```python
from build123d import *

# Parameters (mm, degrees)
SKETCH1_W           = 19
SKETCH1_H           = 81
BOSS_EXTRUDE1_DEPTH = 12.5
SKETCH2_W           = 8.5
SKETCH2_H           = 81
CUT_EXTRUDE1_DEPTH  = 6
SKETCH3_W           = 31.784398885
SKETCH3_H           = 20.084620154
CUT_EXTRUDE2_DEPTH  = 82.482700732
SKETCH4_W           = 27.793270948
SKETCH4_H           = 17.497219338
CUT_EXTRUDE3_DEPTH  = 82.444960882
SKETCH5_W           = 2
SKETCH5_H           = 6.3
BOSS_EXTRUDE2_DEPTH = 6


with BuildPart() as part:
    # Sketch1 → Boss-Extrude1 (new body)
    with BuildSketch(Plane.XY):
        with Locations((-0.214285714, -27.308823529)):
            Rectangle(SKETCH1_W, SKETCH1_H)
    extrude(amount=BOSS_EXTRUDE1_DEPTH)

    # Sketch2 → Cut-Extrude1 (cut)
    with BuildSketch(Plane(origin=(0, 0, 0), x_dir=(-1, 0, 0), z_dir=(0, 0, -1))):
        with Locations((0.214285714, -27.308823529)):
            Rectangle(SKETCH2_W, SKETCH2_H)
    extrude(amount=-CUT_EXTRUDE1_DEPTH, mode=Mode.SUBTRACT)

    # Sketch3 → Cut-Extrude2 (cut, through all)
    with BuildSketch(Plane(origin=(0, -64.772690644, -9.103208009), x_dir=(1, 0, 0), z_dir=(0, -0.9902680687415703, -0.13917310096006574))):
        with Locations((-0.737280551, 17.487835558)):
            Rectangle(SKETCH3_W, SKETCH3_H)
    extrude(amount=CUT_EXTRUDE2_DEPTH, mode=Mode.SUBTRACT)

    # Sketch4 → Cut-Extrude3 (cut, through all)
    with BuildSketch(Plane(origin=(0, 12.138481454, 12.138481454), x_dir=(-1, 0, 0), z_dir=(0, 0.7071067811865464, 0.7071067811865488))):
        with Locations((0.087709147, -6.370587608)):
            Rectangle(SKETCH4_W, SKETCH4_H)
    extrude(amount=CUT_EXTRUDE3_DEPTH, mode=Mode.SUBTRACT)

    # Sketch5 → Boss-Extrude2 (add)
    with BuildSketch(Plane(origin=(0, 13.191176471, 0), x_dir=(1, 0, 0), z_dir=(0, 1, 0))):
        with Locations((-8.714285714, -3.15)):
            Rectangle(SKETCH5_W, SKETCH5_H)
        with Locations((8.285714286, -3.15)):
            Rectangle(SKETCH5_W, SKETCH5_H)
    extrude(amount=BOSS_EXTRUDE2_DEPTH)


solid = part.part
```
Can you work these out from the model? Positions are in its coordinate system, mm. A direction names the side the tool comes from. Round coordinates to 2 decimals unless told otherwise and drop trailing zeros. Order: outer loops, then holes, each group sorted by start corner. A loop starts at its lowest first (then second) coordinate and runs counter-clockwise, first axis right, second up. Notation, with made-up numbers: (85, -19) -> (139, -19) arc R20 cw to (139, 10) -> close; hole circle Ø5 at (-0.75, 48). An arc over 180 degrees is marked (long way). Return JSON: item names as keys, results as strings. Group by question number.
1. If we section it at C-C, the plane y = -54: Write out the boundary of the cut face in (x, z), then the cut area to 4 significant figures.
2. If we section it at D-D, the plane z = 1: Write out the boundary of the cut face in (x, y), then the cut area to 3 significant figures.
3. I need wall thicknesses on line 1 (X direction, y = -28, z = 4.5); line 2 (X direction, y = 15, z = 3); line 3 (Z direction, x = 0.5, y = 0). Which ranges of each line are inside material? Lowest first, please. Write a range as [from, to].
4. We'd pull the mould along X, two halves only. Please class faces 1 (the face through (-7, -24, 0)), 2 (the face through (7.286, 16, 3)), 3 (the face through (-9.714, -25, 6)): released by +X, released by -X, zero draft, split by the parting line, or undercut.
5. If we section it at A-A, the plane z = 4.5: Write out the boundary of the cut face in (x, y), then the cut area to 3 significant figures.
6. If we section it at B-B, the plane x = -8.5: Write out the boundary of the cut face in (y, z).
7. Which directions (+Z, -Z, +X, -X, +Y, -Y) give clear straight access to the entire face, cutting with the end or side of a thin tool? Please do faces 4 (the face through (-4.464, -27, 3)), 5 (the face through (-7.714, 16, 3)), 6 (the face through (-9, 16, 6.3)).
8. Will these pins go through, and if not, where does the flat tip stop? pin 1 (9.5 mm diameter, centred on x = -1, y = -12.5, fed in from -Z); pin 2 (6 mm diameter, centred on x = -5, z = 8, fed in from +Y); pin 3 (0.6 mm diameter, centred on x = 8, y = 15, fed in from +Z).
Output values:
{
 "1": {"outline": "(-9.71, 0) -> (-4.46, 0) -> (-4.46, 6) -> (4.04, 6) -> (4.04, 0) -> (9.29, 0) -> (9.29, 12.5) -> (-9.71, 12.5) -> close", "area": "186.5 mm²"},
 "2": {"outline": "(-9.71, -66.19) -> (-4.46, -66.19) -> (-4.46, 13.19) -> (-7.71, 13.19) -> (-7.71, 19.19) -> (-9.71, 19.19) -> close; (4.04, -66.19) -> (9.29, -66.19) -> (9.29, 19.19) -> (7.29, 19.19) -> (7.29, 13.19) -> (4.04, 13.19) -> close", "area": "858 mm²"},
 "3": {"line 1": "[-9.71, -4.46], [4.04, 9.29]", "line 2": "[-9.71, -7.71], [7.29, 9.29]", "line 3": "[6, 12.5]"},
 "4": {"face 1": "zero draft", "face 2": "undercut", "face 3": "released by -X"},
 "5": {"outline": "(-9.71, -66.68) -> (-4.46, -66.68) -> (-4.46, 13.19) -> (-7.71, 13.19) -> (-7.71, 19.19) -> (-9.71, 19.19) -> close; (4.04, -66.68) -> (9.29, -66.68) -> (9.29, 19.19) -> (7.29, 19.19) -> (7.29, 13.19) -> (4.04, 13.19) -> close", "area": "863 mm²"},
 "6": {"outline": "(-67.81, 12.5) -> (-66.05, 0) -> (19.19, 0) -> (19.19, 6.3) -> (13.19, 6.3) -> (13.19, 11.09) -> (11.78, 12.5) -> close"},
 "7": {"face 4": "-Z, +Y, -Y", "face 5": "+Z, -Z, +Y", "face 6": "+Z, +X, -X, +Y"},
 "8": {"pin 1": "z = 0", "pin 2": "y = 13.19", "pin 3": "z = 6.3"}
}
